from build123d import *

# Parameters (mm, degrees)
EXTRUDE_1_DEPTH = 6
SKETCH_2_R      = 1.5
EXTRUDE_2_DEPTH = 6
EXTRUDE_START   = 6
SKETCH_3_R      = 1.5
EXTRUDE_3_DEPTH = 6


with BuildPart() as part:
    # 草图1 → 凸台-拉伸1 (new body)
    with BuildSketch(Plane(origin=(0, 0, 0), x_dir=(1, 0, 0), z_dir=(0, 1, 0))):
        Polygon((3, 0), (1.5, 2.598076211), (-1.5, 2.598076211), (-3, 0), (-1.5, -2.598076211), (1.5, -2.598076211), align=None)
    extrude(amount=EXTRUDE_1_DEPTH)

    # 草图2 → 凸台-拉伸2 (add)
    with BuildSketch(Plane(origin=(0, 6, 0), x_dir=(1, 0, 0), z_dir=(0, 1, 0))):
        with Locations(Location((0, 0, 0), (0, 0, 270))):
            Circle(SKETCH_2_R)
    extrude(amount=EXTRUDE_2_DEPTH)

    # 草图3 → 凸台-拉伸3 (add)
    with BuildSketch(Plane.XZ.offset(EXTRUDE_START)):
        with Locations(Location((0, 0, 0), (0, 0, 90))):
            Circle(SKETCH_3_R)
    extrude(amount=-EXTRUDE_3_DEPTH)


solid = part.part
The model under review builds one solid part; all positions refer to its coordinate system, in mm. A direction names the side the tool comes from. Round coordinates to 2 decimals unless told otherwise and drop trailing zeros. Loops run counter-clockwise (first coordinate to the right, second up) from the corner with the lowest first, then second, coordinate; pieces in that order, holes last. Notation, with made-up numbers: M 60,73.5 L 113,73.5 A24 cw 113,108.5 Z; hole C 44,-0.75 d3. An arc over 180 degrees is marked long. Answer as CSV lines item,"result". Start each with the question number.
Item 1: For faces 1 (the face through (-2.26, 2.96, 1.28)), 2 (the face through (0.45, 8.96, 1.43)), 3 (the face through (-0.45, -3.04, 1.43)), list the 3-axis set-ups (+Z, -Z, +X, -X, +Y, -Y) from which the entire face can be reached by the end or side of a thin tool; tool diameter is ignored.
Item 2: Consider section A-A (x = 0). Write out the cut boundary in (y, z), then the cut area to 3 significant figures.
Item 3: Wall thickness on line 1 (Y direction, x = -2.7, z = -0.2); line 2 (X direction, y = 10, z = -0.75); line 3 (Z direction, x = 0.9, y = 10.25): over which ranges is each line inside the solid? List them lowest first. Write a range as [from, to].
Item 4: Insertion check: P1, Ø1.5, axis at x = -1.5, y = 7.5, coming from the -Z side; P2, Ø1, axis at x = 0.5, z = 2, coming from the -Y side. Each pin has a flat end and moves straight along its axis. Give the tip position at first contact, or say it passes through.
Item 5: Consider section B-B (z = -1.15). Write out the cut boundary in (x, y), then the cut area to 3 significant figures.
Item 6: Consider section D-D (x = -2.4). Write out the cut boundary in (y, z).
Item 7: Consider section C-C (y = -0.75). Write out the cut boundary in (x, z).
Answer:
1,face 1,"+Z, -X, +Y, -Y"
1,face 2,"+Y"
1,face 3,"-Y"
2,outline,"M -6,-1.5 L 0,-1.5 L 0,-2.6 L 6,-2.6 L 6,-1.5 L 12,-1.5 L 12,1.5 L 6,1.5 L 6,2.6 L 0,2.6 L 0,1.5 L -6,1.5 Z"
2,area,"67.2 mm^2"
3,line 1,"y = [0, 6]"
3,line 2,"x = [-1.3, 1.3]"
3,line 3,"z = [-1.2, 1.2]"
4,P1,"stops at z = -1.3"
4,P2,"stops at y = 0"
5,outline,"M -2.34,0 L -0.96,0 L -0.96,-6 L 0.96,-6 L 0.96,0 L 2.34,0 L 2.34,6 L 0.96,6 L 0.96,12 L -0.96,12 L -0.96,6 L -2.34,6 Z"
5,area,"51.1 mm^2"
6,outline,"M 0,-1.04 L 6,-1.04 L 6,1.04 L 0,1.04 Z"
7,outline,"C 0,0 d3"
